```python
from build123d import *

# Parameters (mm, degrees)
F1_FACE_R = 3.175
F3_R      = 2.356723
F6_W      = 10.16
F6_H      = 2.54
F7_DEPTH  = 2.3876


with BuildPart() as f1:
    # F0 (on Front) → F1 (revolve)
    with BuildSketch(Plane.XZ):
        with BuildLine():
            ThreePointArc((5.715, 3.556), (3.268863, 5.883953), (0, 6.731))
            Line((0, 6.731), (0, -9.144))
            Line((0, -9.144), (3.175, -9.144))
            Line((3.175, -9.144), (3.175, 3.556))
            Line((3.175, 3.556), (5.715, 3.556))
        make_face()
    revolve(axis=Axis((0, 0, -1.2065), (0, 0, -1)))

    # F1_face (on face) → F4 section 0
    with BuildSketch(Plane(origin=(0, 0, -9.144), x_dir=(1, 0, 0), z_dir=(0, 0, -1))):
        Circle(F1_FACE_R)
    # F3 (on offset) → F4 section 1
    with BuildSketch(Plane(origin=(0, 0, -10.16), x_dir=(1, 0, 0), z_dir=(0, 0, -1))):
        Circle(F3_R)
    loft()

    # F6 (on offset) → F7 (cut)
    with BuildSketch(Plane(origin=(0, 0, 6.8834), x_dir=(1, 0, 0), z_dir=(0, 0, -1))):
        Rectangle(F6_W, F6_H)
    extrude(amount=F7_DEPTH, mode=Mode.SUBTRACT)


solid = f1.part
```
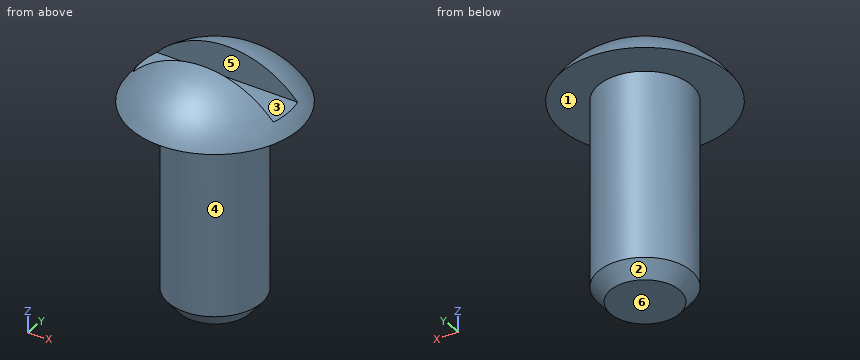
Can you work these out from the model? Positions are in its coordinate system, mm. Face numbers are marked on the shaded views. A direction names the side the tool comes from. Coordinates: 2 decimals unless noted, no trailing zeros. Loops run counter-clockwise (first coordinate to the right, second up) from the corner with the lowest first, then second, coordinate; pieces in that order, holes last. Notation, with made-up numbers: M -32.75,79 L -3.75,79 A11 cw -3.75,85 Z; hole C 84.25,27 d6. An arc over 180 degrees is marked long. Put each result on its own line as item: value. Start each with the question number.
(1) Which directions (+Z, -Z, +X, -X, +Y, -Y) give clear straight access to the entire face, cutting with the end or side of a thin tool? Please do the marked faces 4, 5 and 6.
(2) I need wall thicknesses on probe 1 along Z at (x, y) = (0.5, -0.25); probe 2 along Z at (x, y) = (-4.75, -0.25); probe 3 along Y at (x, z) = (1.5, 6). Which ranges of each line are inside material? Lowest first, please.
(3) Imagine slicing it at A-A on z = -2. List the corners of the cut face in (x, y) for me (3 decimals).
(4) Will these pins go through, and if not, where does the flat tip stop? pin 1 Ø4 at (x, z) = (-1.5, 0.5) entering from +Y (3 decimals); pin 2 Ø4 at (y, z) = (-2, 4) entering from +X; pin 3 Ø0.6 at (x, z) = (2.5, 6) entering from -Y.
(5) We'd pull the mould along Y, two halves only. Please class the marked faces 1, 2 and 3: +Y half, -Y half, draft (parallel to the pull), parting line (faces both ways), or undercut.
Worked answers:
1. face 4: -Z
1. face 5: +Z, +X, -X
1. face 6: -Z, +X, -X, +Y, -Y
2. probe 1: z = -10.16 to 4.5
2. probe 2: z = 3.56 to 4.5
2. probe 3: y = -2.66 to -1.27, 1.27 to 2.66
3. outline: C 0,0 d6.35
4. pin 1: stops at y = 3.175
4. pin 2: stops at x = 5.71
4. pin 3: stops at y = -2.62
5. face 1: draft
5. face 2: parting line
5. face 3: undercut
